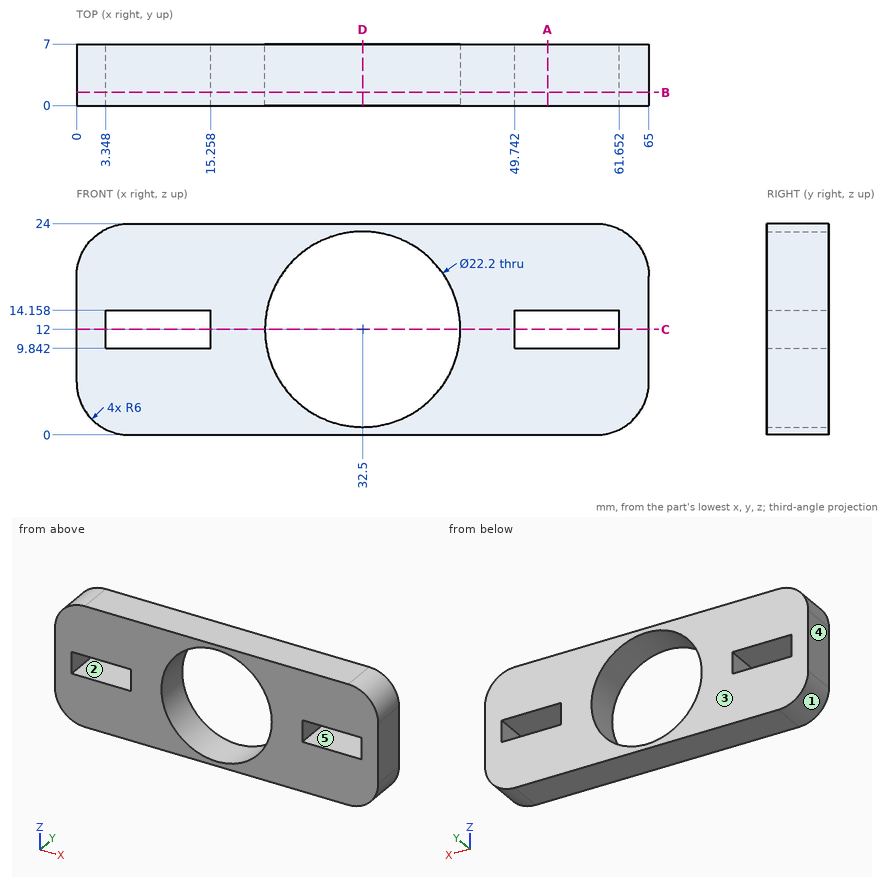
Study the drawing (mm; zero at the part's minimum x, y, z) and answer. A direction names the side the tool comes from. Give positions to 0.01 mm unless a question says otherwise; leave off trailing zeros. Loops run counter-clockwise (first coordinate to the right, second up) from the corner with the lowest first, then second, coordinate; pieces in that order, holes last. Notation, with made-up numbers: (44, -16.5) -> (58, -16.5) arc R13 ccw to (58, 2.5) -> close; hole circle Ø2 at (15.25, 82). An arc over 180 degrees is marked (long way). Use a Markdown table: item, result. Add a question column.
1) The part is cut by section A-A, the plane x = 53.5. Determine the outline of the cut face in (y, z), plus the area to 3 significant figures.
2) The part is cut by section D-D, the plane x = 32.5. Determine the outline of the cut face in (y, z), plus the area to 3 significant figures.
3) Consider line 1 along Z through (x, y) = (12, 6.25); line 2 along Z through (x, y) = (32.5, 4.25); line 3 along X through (y, z) = (2.5, 12.5). Determine where each line is inside the solid, lowest interval first.
4) The part is cut by section C-C, the plane z = 12. Determine the outline of the cut face in (x, y), plus the area to 3 significant figures.
5) Which of the six approach directions +Z, -Z, +X, -X, +Y, -Y give full straight-line access (tool end or side, diameter ignored) to the marked faces 4 and 5?
6) For a pull along X with two mould halves and no side action, classify the marked faces 1, 2 and 3 as +X half, -X half, draft (parallel to the pull), parting line (faces both ways), or undercut.
7) This flat-tipped pin is pushed along its axis until it touches: P1, Ø2, axis at x = 55, y = 3, coming from the -Z side. Where does it stop, or does it pass through?
8) The part is cut by section B-B, the plane y = 1.5. Determine the outline of the cut face in (x, z), plus the area to 3 significant figures.
Reported:
| question | item | result |
|---|---|---|
| 1 | outline | (0, 0) -> (7, 0) -> (7, 9.84) -> (0, 9.84) -> close; (0, 14.16) -> (7, 14.16) -> (7, 24) -> (0, 24) -> close |
| 1 | area | 138 mm^2 |
| 2 | outline | (0, 0) -> (7, 0) -> (7, 0.9) -> (0, 0.9) -> close; (0, 23.1) -> (7, 23.1) -> (7, 24) -> (0, 24) -> close |
| 2 | area | 12.6 mm^2 |
| 3 | line 1 | z = 0 to 9.84, 14.16 to 24 |
| 3 | line 2 | z = 0 to 0.9, 23.1 to 24 |
| 3 | line 3 | x = 0 to 3.35, 15.26 to 21.41, 43.59 to 49.74, 61.65 to 65 |
| 4 | outline | (0, 0) -> (3.35, 0) -> (3.35, 7) -> (0, 7) -> close; (15.26, 0) -> (21.4, 0) -> (21.4, 7) -> (15.26, 7) -> close; (43.6, 0) -> (49.74, 0) -> (49.74, 7) -> (43.6, 7) -> close; (61.65, 0) -> (65, 0) -> (65, 7) -> (61.65, 7) -> close |
| 4 | area | 133 mm^2 |
| 5 | face 4 | +Z, -Z, -X, +Y, -Y |
| 5 | face 5 | +Y, -Y |
| 6 | face 1 | -X half |
| 6 | face 2 | undercut |
| 6 | face 3 | draft |
| 7 | P1 | stops at z = 0 |
| 8 | outline | (0, 6) arc R6 ccw to (6, 0) -> (59, 0) arc R6 ccw to (65, 6) -> (65, 18) arc R6 ccw to (59, 24) -> (6, 24) arc R6 ccw to (0, 18) -> close; hole (3.35, 9.84) -> (15.26, 9.84) -> (15.26, 14.16) -> (3.35, 14.16) -> close; hole circle Ø22.2 at (32.5, 12); hole (49.74, 9.84) -> (61.65, 9.84) -> (61.65, 14.16) -> (49.74, 14.16) -> close |
| 8 | area | 1,040 mm^2 |
